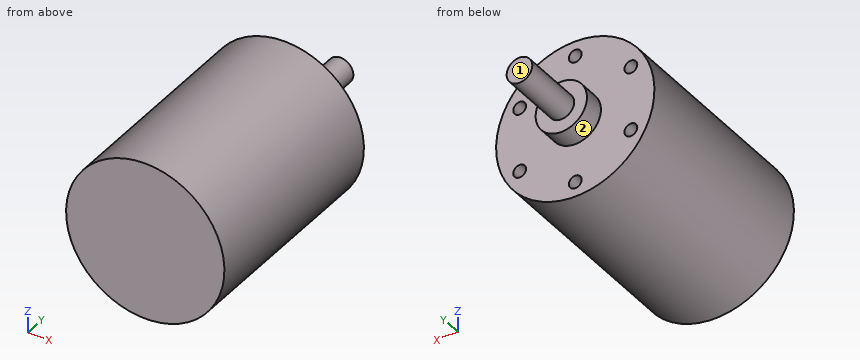
```python
from build123d import *

# Parameters (mm, degrees)
SKETCH1_R           = 18.5
BOSS_EXTRUDE1_DEPTH = 50
SKETCH2_R           = 6
BOSS_EXTRUDE2_DEPTH = 5
SKETCH3_R           = 3
BOSS_EXTRUDE3_DEPTH = 15
SKETCH4_R           = 1.5
CUT_EXTRUDE1_DEPTH  = 10


with BuildPart() as part:
    # Sketch1 → Boss-Extrude1 (new body)
    with BuildSketch(Plane(origin=(0, 0, 0), x_dir=(1, 0, 0), z_dir=(0, 1, 0))):
        with Locations(Location((0, 0, 0), (0, 0, 270))):
            Circle(SKETCH1_R)
    extrude(amount=BOSS_EXTRUDE1_DEPTH)

    # Sketch2 → Boss-Extrude2 (add)
    with BuildSketch(Plane(origin=(0, 50, 0), x_dir=(1, 0, 0), z_dir=(0, 1, 0))):
        with Locations(Location((0, 0, 0), (0, 0, 270))):
            Circle(SKETCH2_R)
    extrude(amount=BOSS_EXTRUDE2_DEPTH)

    # Sketch3 → Boss-Extrude3 (add)
    with BuildSketch(Plane(origin=(0, 55, 0), x_dir=(1, 0, 0), z_dir=(0, 1, 0))):
        with Locations(Location((0, 0, 0), (0, 0, 270))):
            Circle(SKETCH3_R)
    extrude(amount=BOSS_EXTRUDE3_DEPTH)

    # Sketch4 → Cut-Extrude1 (cut)
    with BuildSketch(Plane(origin=(0, 50, 0), x_dir=(1, 0, 0), z_dir=(0, 1, 0))):
        with Locations(Location((0, 15, 0), (0, 0, 270))):
            Circle(SKETCH4_R)
        with Locations(Location((12.990381057, 7.5, 0), (0, 0, 270))):
            Circle(SKETCH4_R)
        with Locations(Location((12.990381057, -7.5, 0), (0, 0, 270))):
            Circle(SKETCH4_R)
        with Locations(Location((0, -15, 0), (0, 0, 270))):
            Circle(SKETCH4_R)
        with Locations(Location((-12.990381057, -7.5, 0), (0, 0, 270))):
            Circle(SKETCH4_R)
        with Locations(Location((-12.990381057, 7.5, 0), (0, 0, 270))):
            Circle(SKETCH4_R)
    extrude(amount=-CUT_EXTRUDE1_DEPTH, mode=Mode.SUBTRACT)


solid = part.part
```
Part model, mm, in its own coordinate system. Face numbers are marked on the shaded views. A direction names the side the tool comes from. Give positions to 0.01 mm unless a question says otherwise; leave off trailing zeros. Order: outer loops, then holes, each group sorted by start corner. A loop starts at its lowest first (then second) coordinate and runs counter-clockwise, first axis right, second up. Notation, with made-up numbers: M 23,43.5 L 64,43.5 A21 cw 64,67.5 Z; hole C 89,-12 d10. An arc over 180 degrees is marked long. Use a Markdown table: item, result. Add a question column.
(1) Drop flat-ended pins along their axis: P1, Ø3.5, axis at x = -12.5, z = -8, coming from the +Y side; P2, Ø12, axis at x = -14.5, y = 36.5, coming from the -Z side; P3, Ø8, axis at x = 14.5, y = 20, coming from the +Z side. Give the stop position or say it passes through.
(2) Saw through at C-C, the plane y = 16. Give the cut face in (x, z), and give its area (3 significant figures).
(3) Saw through at B-B, the plane z = 7.5. Give the cut face in (x, y).
(4) 3-axis set-ups, long thin cutter, end or side, ignore diameter. For the marked faces 1 and 2: which of +Z, -Z, +X, -X, +Y, -Y reach the whole face in a straight line?
(5) Saw through at A-A, the plane y = 41.5. Give the cut face in (x, z), and give its area (3 significant figures).
(6) Probe line 1 along X through (y, z) = (42.25, 7.5); line 2 along X through (y, z) = (42, 7); line 3 along Y through (x, z) = (4, 1.5). List the from-to ranges inside material, lowest first. Write a range as [from, to].
(7) Saw through at D-D, the plane x = 8.5. Give the cut face in (y, z).
Answer key:
| question | item | result |
|---|---|---|
| 1 | P1 | y = 50 |
| 1 | P2 | z = -16.43 |
| 1 | P3 | z = 15.23 |
| 2 | outline | C 0,0 d37 |
| 2 | area | 1,080 mm^2 |
| 3 | outline | M -16.91,0 L 16.91,0 L 16.91,50 L 14.49,50 L 14.49,40 L 11.49,40 L 11.49,50 L -11.49,50 L -11.49,40 L -14.49,40 L -14.49,50 L -16.91,50 Z |
| 4 | face 1 | +Z, -Z, +X, -X, +Y |
| 4 | face 2 | +Y |
| 5 | outline | C 0,0 d37; hole C -12.99,-7.5 d3; hole C -12.99,7.5 d3; hole C 0,-15 d3; hole C 0,15 d3; hole C 12.99,-7.5 d3; hole C 12.99,7.5 d3 |
| 5 | area | 1,030 mm^2 |
| 6 | line 1 | [-16.91, -14.49], [-11.49, 11.49], [14.49, 16.91] |
| 6 | line 2 | [-17.12, -14.4], [-11.58, 11.58], [14.4, 17.12] |
| 6 | line 3 | [0, 55] |
| 7 | outline | M 0,-16.43 L 50,-16.43 L 50,16.43 L 0,16.43 Z |
